Work out the finished part from the listing and answer in its coordinate system (mm). A direction names the side the tool comes from. Coordinates: 2 decimals unless noted, no trailing zeros. Loops run counter-clockwise (first coordinate to the right, second up) from the corner with the lowest first, then second, coordinate; pieces in that order, holes last. Notation, with made-up numbers: (74, -28.5) - (79, -28.5) arc R20 cw to (79, -22.5) - close; hole circle Ø11 at (53.5, 29). An arc over 180 degrees is marked (long way). Write each question's results on one line, items separated by ' | '. Start each with the question number.
Item 1: Each of these flat-tipped pins is pushed along its axis until it touches: pin 1 Ø0.9 at (y, z) = (0, -0.5) entering from -X; pin 2 Ø6 at (x, z) = (80, 0) entering from +Y; pin 3 Ø1.5 at (y, z) = (0, -3.5) entering from -X. Where does it stop, or does it pass through?
Item 2: Section D-D, the plane z = 4.5 is taken. Write down the section's boundary in (x, y), plus the area to 3 significant figures.
Item 3: Consider probe 1 along Z at (x, y) = (0, 0.75); probe 2 along X at (y, z) = (1, 1); probe 3 along Z at (x, y) = (14, 1.1). Determine where each line is inside the solid, lowest interval first. Write a range as [from, to].
Item 4: For a pull along X with two mould halves and no side action, classify faces 3 (the face through (68, 0, -0.75)), 4 (the face through (-6, 0, 0)), 5 (the face through (78.339, -0.021, 3.194)), 6 (the face through (41, 1.5, 0)) as +X half, -X half, draft (parallel to the pull), parting line (faces both ways), or undercut.
Item 5: Section B-B, the plane x = 10.5 is taken. Write down the section's boundary in (y, z), plus the area to 3 significant figures.
Item 6: Section C-C, the plane y = 0.85 is taken. Write down the section's boundary in (x, z), plus the area to 3 significant figures.
Item 7: A tool of negligible diameter and unlimited length cuts with its end or side. For faces 1 (the face through (41, 0, -6)), 2 (the face through (18, 0, 0)), from which of +Z, -Z, +X, -X, +Y, -Y can it reach the whole face along a straight path? Write none if from no direction.
Item 8: Section A-A, the plane z = 0 is taken. Write down the section's boundary in (x, y).
Autodesk Inventor part; units mm, degrees
ref_plane "YZ Plane" through (0, 0, 0) normal (1, 0, 0) x (0, 1, 0)
ref_plane "XZ Plane" through (0, 0, 0) normal (0, 1, 0) x (-1, 0, 0)
ref_plane "XY Plane" through (0, 0, 0) normal (0, 0, 1) x (1, 0, 0)
sketch "草圖1" plane through (0, 0, 0) normal (0, 1, 0) x (-1, 0, 0)
  circle A0 centre (0, 0) radius 1.25
  line L0 (0, 0) -> (-80, 0)
  circle A1 centre (-80, 0) radius 3.6
  circle A2 centre (-80, 0) radius 6
  circle A3 centre (0, 0) radius 6
  line L1 (0, 6) -> (-80, 6)
  line L2 (-80, -6) -> (0, -6)
  dimension "d0" = 2.5
  dimension "d14" = 80
  dimension "d15" = 7.2
  dimension "d16" = 12
  dimension "d17" = 12
extrude "擠出1" add sketch "草圖1" along normal mid plane 3
sketch "草圖2" plane through (0, 1.5, 0) normal (0, 1, 0) x (1, 0, 0)
  circle A0 centre (80, 0) radius 3.6
  circle A1 centre (0, 0) radius 1.25
  arc A2 (0, 6) -> (0, -6) centre (0, 0) ccw
  line L0 (0, -6) -> (80, -6)
  arc A3 (80, -6) -> (80, 6) centre (80, 0) ccw
  line L1 (80, 6) -> (0, 6)
  line L2 (80, 0) -> (70, 0)
  line L3 (70, 0) -> (65, 0) construction
  line L4 (70, 0.75) -> (65, 0.75)
  line L5 (65, -0.75) -> (70, -0.75)
  arc A4 (70, -0.75) -> (70, 0.75) centre (70, 0) ccw
  arc A5 (65, 0.75) -> (65, -0.75) centre (65, 0) ccw
  line L6 (65, 0) -> (57, 0)
  line L7 (57, 0) -> (57, 1.5)
  line L8 (57, 1.5) -> (48, 1.5)
  line L9 (48, 1.5) -> (48, -1.5)
  line L10 (48, -1.5) -> (57, -1.5)
  line L11 (57, -1.5) -> (57, 0)
  line L12 (48, 0) -> (32, 0)
  circle A6 centre (32, 0) radius 1.5
  line L13 (32, 0) -> (18, 0)
  line L14 (18, 0) -> (18, 1.5)
  line L15 (18, 1.5) -> (9, 1.5)
  line L16 (9, 1.5) -> (9, -1.5)
  line L17 (9, -1.5) -> (18, -1.5)
  line L18 (18, -1.5) -> (18, 0)
  point P0 (67.5, 0)
  dimension "d18" = 10
  dimension "d19" = 5
  dimension "d20" = 1.5
  dimension "d21" = 8
  dimension "d22" = 1.5
  dimension "d23" = 9
  dimension "d24" = 3
  dimension "d25" = 16
  dimension "d27" = 3
  dimension "d28" = 14
  dimension "d29" = 1.5
  dimension "d30" = 9
  dimension "d31" = 3
extrude "擠出2" cut sketch "草圖2" against normal blind 10 contours L18 L17 L16 L15 L14 | A6 L13 L12 | L12 L13 A6 | L11 L10 L9 L8 L7 | A4 L5 A5 L4
properties part number "連接3"
Answer key:
1) pin 1: stops at x = -6 | pin 2: passes through | pin 3: stops at x = -5.33
2) outline: (-3.97, -1.5) - (83.97, -1.5) - (83.97, 1.5) - (-3.97, 1.5) - close | area: 264 mm^2
3) probe 1: z = [-6, -1.25], [1.25, 6] | probe 2: x = [-5.92, -0.75], [0.75, 9], [18, 30.88], [33.12, 48], [57, 76.54], [83.46, 85.92] | probe 3: z = [-6, -1.5], [1.5, 6]
4) face 3: undercut | face 4: -X half | face 5: undercut | face 6: draft
5) outline: (-1.5, -6) - (1.5, -6) - (1.5, -1.5) - (-1.5, -1.5) - close; (-1.5, 1.5) - (1.5, 1.5) - (1.5, 6) - (-1.5, 6) - close | area: 27.0 mm^2
6) outline: (0, -6) - (80, -6) arc R6 ccw to (80, 6) - (0, 6) arc R6 ccw to start; hole circle Ø2.5 at (0, 0); hole (9, -1.5) - (18, -1.5) - (18, 1.5) - (9, 1.5) - close; hole circle Ø3 at (32, 0); hole (48, -1.5) - (57, -1.5) - (57, 1.5) - (48, 1.5) - close; hole (65, -0.75) - (70, -0.75) arc R0.75 ccw to (70, 0.75) - (65, 0.75) arc R0.75 ccw to start; hole circle Ø7.2 at (80, 0) | area: 957 mm^2
7) face 1: -Z, +X, -X, +Y, -Y | face 2: +Y, -Y
8) outline: (-6, -1.5) - (-1.25, -1.5) - (-1.25, 1.5) - (-6, 1.5) - close; (1.25, -1.5) - (9, -1.5) - (9, 1.5) - (1.25, 1.5) - close; (18, -1.5) - (30.5, -1.5) - (30.5, 1.5) - (18, 1.5) - close; (33.5, -1.5) - (48, -1.5) - (48, 1.5) - (33.5, 1.5) - close; (57, -1.5) - (64.25, -1.5) - (64.25, 1.5) - (57, 1.5) - close; (70.75, -1.5) - (76.4, -1.5) - (76.4, 1.5) - (70.75, 1.5) - close; (83.6, -1.5) - (86, -1.5) - (86, 1.5) - (83.6, 1.5) - close
